```python
from build123d import *

# Parameters (mm, degrees)
SKETCH1_R               = 7.5
BOSS_EXTRUDE1_DEPTH     = 58
CUT_EXTRUDE1_DEPTH      = 58
SKETCH4_R               = 7
CUT_EXTRUDE2_DEPTH      = 58
CUT_EXTRUDE3_DEPTH      = 96.859271852
CUT_EXTRUDE3_DEPTH_BACK = 6
SKETCH5_R               = 7.5
CUT_EXTRUDE5_START      = -6
CUT_EXTRUDE5_DEPTH      = 6
CUT_EXTRUDE6_DEPTH      = 6
CUT_EXTRUDE7_DEPTH      = 6


with BuildPart() as part:
    # Sketch1 → Boss-Extrude1 (new body)
    with BuildSketch(Plane.XY):
        with BuildLine():
            Line((0, 0), (-65, 0))
            Line((-65, 0), (-65, 24))
            ThreePointArc((-65, 24), (-50.249936753, 35.04674653), (-32.5, 40))
            Line((-32.5, 40), (0, 40))
            Line((0, 40), (15, 31.339745962))
            Line((15, 31.339745962), (15, 8.660254038))
            Line((15, 8.660254038), (0, 0))
        make_face()
        with Locations((-31, 19)):
            Circle(SKETCH1_R, mode=Mode.SUBTRACT)
    extrude(amount=-BOSS_EXTRUDE1_DEPTH)

    # Sketch3 → Cut-Extrude1 (cut)
    with BuildSketch(Plane(origin=(0, 40, 0), x_dir=(1, 0, 0), z_dir=(0, 1, 0))):
        Polygon((-65, 50), (-49, 50), (-49, 44), (-11, 44), (-11, 14), (-49, 14), (-49, 8), (-65, 8), align=None)
        Polygon((0, 58), (15, 43), (15, 58), align=None)
        Polygon((0, 0), (15, 15), (15, 0), align=None)
    extrude(amount=-CUT_EXTRUDE1_DEPTH, mode=Mode.SUBTRACT)

    # Sketch4 → Cut-Extrude2 (cut)
    with BuildSketch(Plane(origin=(15, 0, 0), x_dir=(0, 0, -1), z_dir=(1, 0, 0))):
        with Locations(Location((29, 20, 0), (0, 0, 90))):
            Circle(SKETCH4_R)
    extrude(amount=-CUT_EXTRUDE2_DEPTH, mode=Mode.SUBTRACT)

    # Sketch5 → Cut-Extrude3 (cut, two sides: drawn at the far end of the back side and taken through both)
    with BuildSketch(Plane.XY.offset(-CUT_EXTRUDE3_DEPTH_BACK)):
        with BuildLine():
            Line((-65, 22), (-65, 2))
            Line((-65, 2), (-2, 2))
            Line((-2, 2), (-2, 38))
            Line((-2, 38), (-32.5, 38))
            ThreePointArc((-32.5, 38), (-50.249936753, 33.04674653), (-65, 22))
        make_face()
        with Locations((-31, 19)):
            Circle(SKETCH5_R, mode=Mode.SUBTRACT)
    extrude(amount=CUT_EXTRUDE3_DEPTH + CUT_EXTRUDE3_DEPTH_BACK, mode=Mode.SUBTRACT)

    # Sketch7 → Cut-Extrude5 (cut)
    with BuildSketch(Plane.XY.offset(-6).offset(CUT_EXTRUDE5_START)):
        with BuildLine():
            Line((-47, 34.505277409), (-47, 2))
            Line((-47, 2), (-2, 2))
            Line((-2, 2), (-2, 38))
            Line((-2, 38), (-32.5, 38))
            ThreePointArc((-32.5, 38), (-39.881044096, 36.796355507), (-47, 34.505277409))
        make_face()
    extrude(amount=CUT_EXTRUDE5_DEPTH, mode=Mode.SUBTRACT)

    # Sketch8 → Cut-Extrude6 (cut)
    with BuildSketch(Plane(origin=(0, 0, -58), x_dir=(-1, 0, 0), z_dir=(0, 0, -1))):
        with BuildLine():
            Line((2, 2), (65, 2))
            Line((65, 2), (65, 22))
            ThreePointArc((65, 22), (50.249936753, 33.04674653), (32.5, 38))
            Line((32.5, 38), (2, 38))
            Line((2, 38), (2, 2))
        make_face()
    extrude(amount=-CUT_EXTRUDE6_DEPTH, mode=Mode.SUBTRACT)

    # Sketch9 → Cut-Extrude7 (cut)
    with BuildSketch(Plane(origin=(0, 0, -52), x_dir=(-1, 0, 0), z_dir=(0, 0, -1))):
        with BuildLine():
            Line((47, 34.505277409), (47, 2))
            Line((47, 2), (2, 2))
            Line((2, 2), (2, 38))
            Line((2, 38), (32.5, 38))
            ThreePointArc((32.5, 38), (39.881044096, 36.796355507), (47, 34.505277409))
        make_face()
    extrude(amount=-CUT_EXTRUDE7_DEPTH, mode=Mode.SUBTRACT)


solid = part.part
```
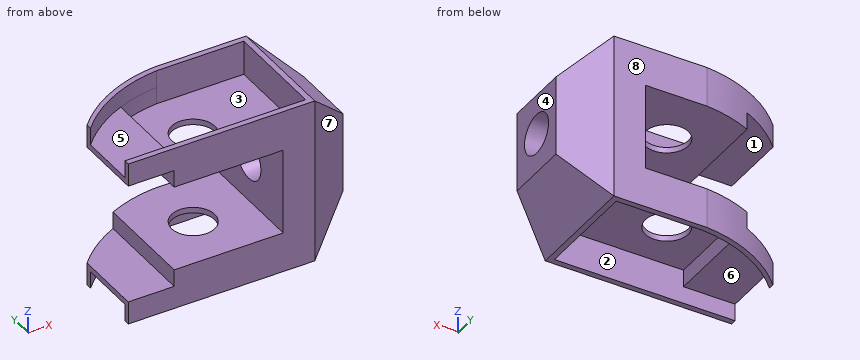
The listing builds one solid part. Answer for the finished solid, in the listing's coordinates (mm). Face numbers are marked on the shaded views. A direction names the side the tool comes from. Round coordinates to 2 decimals unless told otherwise and drop trailing zeros. Loops run counter-clockwise (first coordinate to the right, second up) from the corner with the lowest first, then second, coordinate; pieces in that order, holes last. Notation, with made-up numbers: (-35, 5.25) -> (19, 5.25) arc R24 cw to (19, 20.25) -> close; hole circle Ø8 at (22.5, 14). An arc over 180 degrees is marked (long way). Use one line per item in the form item = value.
1. The part is cut by section D-D on y = 19. Give the number of separate pieces and of enclosed holes in the cut face, and give its area (3 significant figures).
Answer key:
separate_pieces = 4
enclosed_holes = 0
area = 887 mm²
2. The part is cut by section C-C on x = -57.5. Determine the outline of the cut face in (y, z), and give its area (3 significant figures).
Answer key:
outline = (0, -58) -> (2, -58) -> (2, -52) -> (28.68, -52) -> (28.68, -58) -> (30.68, -58) -> (30.68, -50) -> (0, -50) -> close; (0, -8) -> (30.68, -8) -> (30.68, 0) -> (28.68, 0) -> (28.68, -6) -> (2, -6) -> (2, 0) -> (0, 0) -> close
area = 171 mm²
3. The part is cut by section A-A on x = -31. Determine the outline of the cut face in (y, z), and give its area (3 significant figures).
Answer key:
outline = (0, -58) -> (2, -58) -> (2, -46) -> (11.5, -46) -> (11.5, -44) -> (0, -44) -> close; (0, -14) -> (11.5, -14) -> (11.5, -12) -> (2, -12) -> (2, 0) -> (0, 0) -> close; (26.5, -46) -> (38, -46) -> (38, -58) -> (40, -58) -> (40, -44) -> (26.5, -44) -> close; (26.5, -14) -> (40, -14) -> (40, 0) -> (38, 0) -> (38, -12) -> (26.5, -12) -> close
area = 196 mm²
4. For a pull along Y with two mould halves and no side action, classify the marked faces 5, 6, 7 and 8 as released by +Y, released by -Y, zero draft, split by the parting line, or undercut.
Answer key:
face_5 = undercut
face_6 = undercut
face_7 = released by -Y
face_8 = released by +Y
5. Flat-ended cylindrical pins translate along their axes: pin 1 Ø8 at (x, y) = (-59.5, 14.5) entering from +Z; pin 2 Ø24 at (x, y) = (-31, 19) entering from +Z; pin 3 Ø6 at (x, y) = (4, 8.5) entering from -Z. Find the tip coordinate at first contact, or state that the pin passes through.
Answer key:
pin_1 = -6
pin_2 = -12
pin_3 = -57
6. The part is cut by section B-B on z = -29. Determine the outline of the cut face in (x, y).
Answer key:
outline = (-11, 0) -> (0, 0) -> (15, 8.66) -> (15, 13) -> (-11, 13) -> close; (-11, 27) -> (15, 27) -> (15, 31.34) -> (0, 40) -> (-11, 40) -> close
7. Find the intervals of material crossed by probe 1 along Z at (x, y) = (-40, 25.5); probe 2 along Z at (x, y) = (-0.75, 20); probe 3 along Y at (x, z) = (-31, -45), in increasing order. Write a range as [from, to].
Answer key:
probe_1 = [-46, -44], [-14, -12]
probe_2 = [-58, -36], [-22, 0]
probe_3 = [0, 11.5], [26.5, 40]
8. A tool of negligible diameter and unlimited length cuts with its end or side. For the marked faces 1, 2, 3 and 4, from which of +Z, -Z, +X, -X, +Y, -Y can it reach the whole face along a straight path? Write none if from no direction.
Answer key:
face_1 = -X, +Y, -Y
face_2 = -Z
face_3 = +Z
face_4 = +Z, -Z, +X, +Y, -Y
